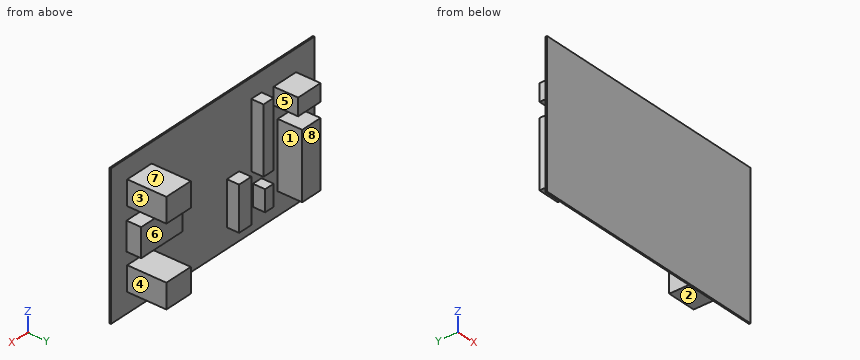
```python
from build123d import *

# Parameters (mm, degrees)
SKETCH1_W           = 500
SKETCH1_H           = 290
BOSS_EXTRUDE1_DEPTH = 3
SKETCH3_W           = 60
SKETCH3_H           = 50
BOSS_EXTRUDE2_DEPTH = 80
SKETCH4_W           = 102
SKETCH4_H           = 58
BOSS_EXTRUDE3_DEPTH = 30
SKETCH5_W           = 30
SKETCH5_H           = 90
SKETCH5_W_2         = 21
SKETCH5_H_2         = 43.2
SKETCH5_W_3         = 25
SKETCH5_H_3         = 135
BOSS_EXTRUDE4_DEPTH = 25
SKETCH6_W           = 55
SKETCH6_H           = 35
SKETCH6_W_2         = 45
SKETCH6_H_2         = 135
BOSS_EXTRUDE5_DEPTH = 50


with BuildPart() as part:
    # Sketch1 → Boss-Extrude1 (new body)
    with BuildSketch(Plane(origin=(0, 0, 0), x_dir=(1, 0, 0), z_dir=(0, 1, 0))):
        with Locations((250, 145)):
            Rectangle(SKETCH1_W, SKETCH1_H)
    extrude(amount=BOSS_EXTRUDE1_DEPTH)

    # Sketch3 → Boss-Extrude2 (add)
    with BuildSketch(Plane(origin=(0, 3, 0), x_dir=(1, 0, 0), z_dir=(0, 1, 0))):
        with Locations((430, 225)):
            Rectangle(SKETCH3_W, SKETCH3_H)
        with Locations((430, 65)):
            Rectangle(SKETCH3_W, SKETCH3_H)
    extrude(amount=BOSS_EXTRUDE2_DEPTH)

    # Sketch4 → Boss-Extrude3 (add)
    with BuildSketch(Plane(origin=(0, 3, 0), x_dir=(1, 0, 0), z_dir=(0, 1, 0))):
        with Locations((410.73324546, 145)):
            Rectangle(SKETCH4_W, SKETCH4_H)
    extrude(amount=BOSS_EXTRUDE3_DEPTH)

    # Sketch5 → Boss-Extrude4 (add)
    with BuildSketch(Plane(origin=(0, 3, 0), x_dir=(1, 0, 0), z_dir=(0, 1, 0))):
        with Locations((200, 205)):
            Rectangle(SKETCH5_W, SKETCH5_H)
        with Locations((140.5, 221.6)):
            Rectangle(SKETCH5_W_2, SKETCH5_H_2)
        with Locations((142.5, 107.5)):
            Rectangle(SKETCH5_W_3, SKETCH5_H_3)
    extrude(amount=BOSS_EXTRUDE4_DEPTH)

    # Sketch6 → Boss-Extrude5 (add)
    with BuildSketch(Plane(origin=(0, 3, 0), x_dir=(1, 0, 0), z_dir=(0, 1, 0))):
        with Locations((72.5, 61.564484871)):
            Rectangle(SKETCH6_W, SKETCH6_H)
        with Locations((67.5, 176.564484871)):
            Rectangle(SKETCH6_W_2, SKETCH6_H_2)
    extrude(amount=BOSS_EXTRUDE5_DEPTH)


solid = part.part
```
Design review of the part built by this model. Coordinates are the model's own, in mm. Face numbers are marked on the shaded views. A direction names the side the tool comes from. Give positions to 0.01 mm unless a question says otherwise; leave off trailing zeros. Loops run counter-clockwise (first coordinate to the right, second up) from the corner with the lowest first, then second, coordinate; pieces in that order, holes last. Notation, with made-up numbers: M 42,78 L 76,78 A24 ccw 76,101 Z; hole C 75.25,77 d6. An arc over 180 degrees is marked long. Return JSON: item names as keys, results as strings. Group by question number.
Item 1: We need section A-A (y = 76.5). Give the boundary of the cut face in (x, z).
Item 2: We need section D-D (z = -51.5). Give the boundary of the cut face in (x, y).
Item 3: Tool access review of the marked faces 4, 5, 6, 7 and 8: name each direction out of +Z, -Z, +X, -X, +Y, -Y from which nothing blocks a thin tool from reaching the whole face with its end or side.
Item 4: Insertion check: pin 1 Ø3 at (y, z) = (8.5, -167) entering from +X; pin 2 Ø12.5 at (x, y) = (137, 9.5) entering from -Z; pin 3 Ø18 at (x, y) = (428, 31.5) entering from +Z. Each pin has a flat end and moves straight along its axis. Give the tip position at first contact, or say it passes through.
Item 5: For probe 1 along X at (y, z) = (21, -219); probe 2 along Z at (x, y) = (435.5, 33.5); probe 3 along X at (y, z) = (6.5, -109.5), list the stretches that pass through material, from the lowest coordinate up.
Item 6: We need section B-B (x = 365). Give the boundary of the cut face in (y, z), and give its area (3 significant figures).
Item 7: We need section C-C (z = -137). Give the boundary of the cut face in (x, y), and give its area (4 significant figures).
Item 8: Mouldability with a two-part tool opening along X and no side actions: class the marked faces 1, 2 and 3 as released by +X, released by -X, zero draft, split by the parting line, or undercut.
Output:
{
 "1": {"outline": "M 400,-250 L 460,-250 L 460,-200 L 400,-200 Z; M 400,-90 L 460,-90 L 460,-40 L 400,-40 Z"},
 "2": {"outline": "M 0,0 L 500,0 L 500,3 L 460,3 L 460,83 L 400,83 L 400,3 L 155,3 L 155,28 L 130,28 L 130,3 L 100,3 L 100,53 L 45,53 L 45,3 L 0,3 Z"},
 "3": {"face 4": "-Z, +X, +Y", "face 5": "+Z, -Z, +Y", "face 6": "+X, +Y", "face 7": "+Z, +X, -X, +Y", "face 8": "+Z, -Z, -X, +Y"},
 "4": {"pin 1": "stops at x = 461.73", "pin 2": "stops at z = -243.2", "pin 3": "stops at z = -40"},
 "5": {"probe 1": "x = 45 to 90, 130 to 151, 185 to 215, 400 to 460", "probe 2": "z = -250 to -200, -90 to -40", "probe 3": "x = 45 to 90, 130 to 155"},
 "6": {"outline": "M 0,-290 L 3,-290 L 3,-174 L 33,-174 L 33,-116 L 3,-116 L 3,0 L 0,0 Z", "area": "2,610 mm^2"},
 "7": {"outline": "M 0,0 L 500,0 L 500,3 L 461.73,3 L 461.73,33 L 359.73,33 L 359.73,3 L 155,3 L 155,28 L 130,28 L 130,3 L 90,3 L 90,53 L 45,53 L 45,3 L 0,3 Z", "area": "7,435 mm^2"},
 "8": {"face 1": "undercut", "face 2": "zero draft", "face 3": "released by +X"}
}
